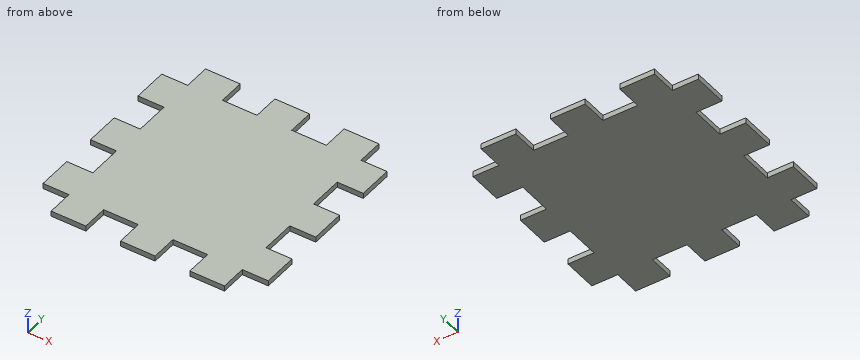
```python
from build123d import *

# Parameters (mm, degrees)
F0_W     = 7.62
F0_H     = 10.16
F0_W_2   = 10.16
F0_H_2   = 7.62
F0_W_3   = 10.160000307
F0_W_4   = 7.619999693
F1_DEPTH = 1.5875


# Not quite as in the source:
# - ends of sketch curves that miss each other by under 0.0002 mm in the source are joined


with BuildPart() as f1:
    # F0 (on Top) → F1 (new body)
    with BuildSketch(Plane.XY):
        with Locations((29.21, -20.32)):
            Rectangle(F0_W, F0_H)
        with Locations((20.320000307, -29.21)):
            Rectangle(F0_W_2, F0_H_2)
        with Locations((3.07e-07, -29.21)):
            Rectangle(F0_W_2, F0_H_2)
        with Locations((-20.3199998465, -29.21)):
            Rectangle(F0_W_3, F0_H_2)
        with Locations((-29.2099998465, -20.32)):
            Rectangle(F0_W_4, F0_H)
        with Locations((-29.2099998465, 0)):
            Rectangle(F0_W_4, F0_H)
        with Locations((-29.2099998465, 20.32)):
            Rectangle(F0_W_4, F0_H)
        with Locations((-20.320000307, 29.21)):
            Rectangle(F0_W_2, F0_H_2)
        with Locations((-3.07e-07, 29.21)):
            Rectangle(F0_W_2, F0_H_2)
        with Locations((20.3199998465, 29.21)):
            Rectangle(F0_W_3, F0_H_2)
        with Locations((29.21, 20.32)):
            Rectangle(F0_W, F0_H)
        Polygon((25.4, 15.24), (25.4, 25.4), (15.239999693, 25.4), (5.079999693, 25.4), (-5.080000307, 25.4), (-15.240000307, 25.4), (-25.4, 25.4), (-25.4, 15.24), (-25.4, 5.08), (-25.4, -5.08), (-25.4, -15.24), (-25.4, -25.4), (-15.239999693, -25.4), (-5.079999693, -25.4), (5.080000307, -25.4), (15.240000307, -25.4), (25.4, -25.4), (25.4, -15.24), (25.4, -5.08), (25.4, 5.08), align=None)
        with Locations((29.21, 0)):
            Rectangle(F0_W, F0_H)
    extrude(amount=F1_DEPTH)


solid = f1.part
```
Check sheet for the modelled part. Datum: model origin and axes. Units: mm. Round coordinates to 2 decimals unless told otherwise and drop trailing zeros. Loops run counter-clockwise (first coordinate to the right, second up) from the corner with the lowest first, then second, coordinate; pieces in that order, holes last. Notation, with made-up numbers: (76, 72) - (81, 72) arc R19 ccw to (81, 89) - close; hole circle Ø6 at (55, -31.75). An arc over 180 degrees is marked (long way). Write item = value, one per line. Start each with the question number.
Q1. Thickness scan on L1, parallel to X at y = -27.5, z = 0.5; L2, parallel to X at y = -12, z = 0.7. Record the ranges inside material, lowest first.
Q2. Section check C-C (x = -14). Record the boundary of the cut face in (y, z), plus the area to 3 significant figures.
Q3. Depth check by flat-ended pin: P1, Ø0.8, axis at y = 8.5, z = 1, coming from the -X side; P2, Ø0.8, axis at x = 28, z = 0.5, coming from the -Y side; P3, Ø0.5, axis at y = -12, z = 1, coming from the +X side. Enter the tip coordinate at first touch or a pass-through.
Q4. Section check A-A (y = -26.5). Record the boundary of the cut face in (x, z).
Derived:
q1.L1 = -25.4 to -15.24, -5.08 to 5.08, 15.24 to 25.4
q1.L2 = -25.4 to 25.4
q2.outline = (-25.4, 0) - (25.4, 0) - (25.4, 1.59) - (-25.4, 1.59) - close
q2.area = 80.6 mm^2
q3.P1 = -25.4
q3.P2 = -25.4
q3.P3 = 25.4
q4.outline = (-25.4, 0) - (-15.24, 0) - (-15.24, 1.59) - (-25.4, 1.59) - close; (-5.08, 0) - (5.08, 0) - (5.08, 1.59) - (-5.08, 1.59) - close; (15.24, 0) - (25.4, 0) - (25.4, 1.59) - (15.24, 1.59) - close
